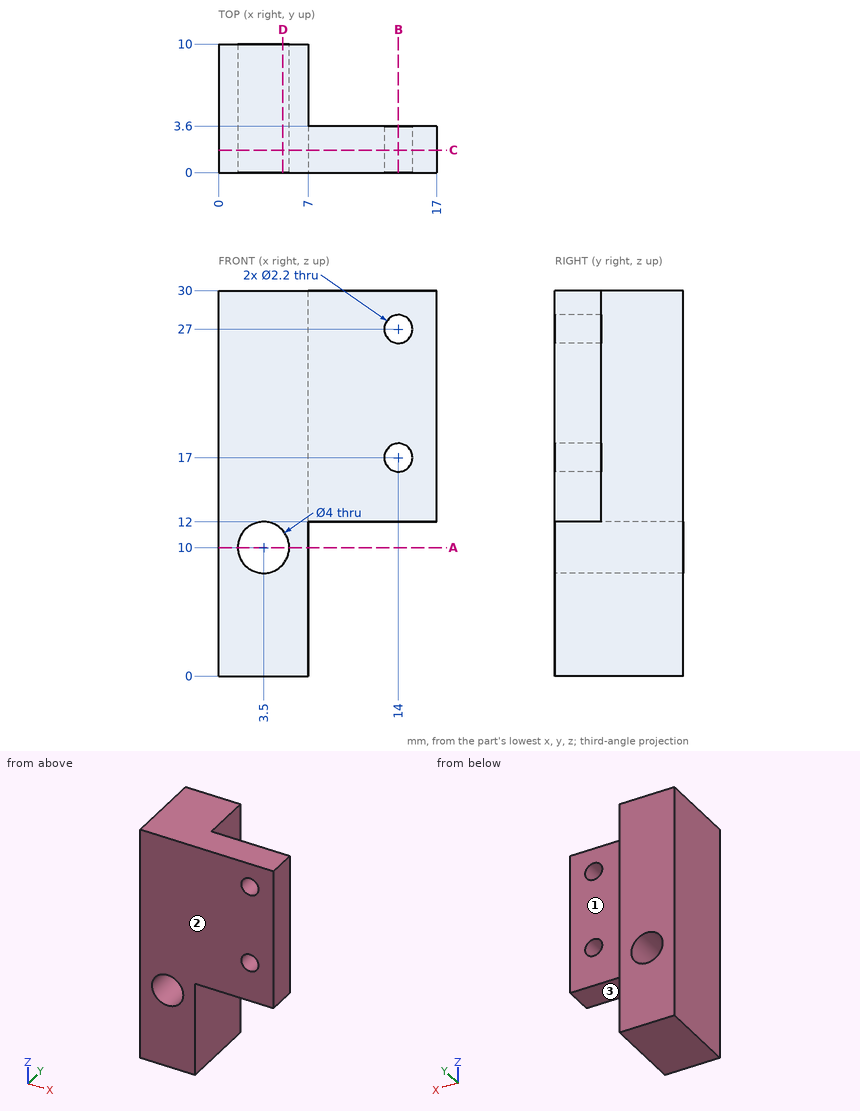
Verification items for this drawing (mm, ordinates from the low corner). A direction names the side the tool comes from. Coordinates: 2 decimals unless noted, no trailing zeros. Order: outer loops, then holes, each group sorted by start corner. A loop starts at its lowest first (then second) coordinate and runs counter-clockwise, first axis right, second up. Notation, with made-up numbers: (-8.75, -11.75) - (28.25, -11.75) arc R31 cw to (28.25, 23.25) - close; hole circle Ø4 at (23.5, 87.5). An arc over 180 degrees is marked (long way). Answer as a JSON object with one key per item and string values. Group by question number.
Item 1: Sectioned sample at D-D, the plane x = 5. Record the cut outline in (y, z), and give its area (3 significant figures).
Item 2: Scan lines: probe 1 along Z at (x, y) = (14, 2.2); probe 2 along Z at (x, y) = (3.5, 5.5); probe 3 along X at (y, z) = (6, 22.75). Record each from-to range of solid material in increasing order.
Item 3: Sectioned sample at C-C, the plane y = 1.75. Record the cut outline in (x, z), and give its area (3 significant figures).
Item 4: Sectioned sample at B-B, the plane x = 14. Record the cut outline in (y, z).
Item 5: Tool access check on the marked faces 1, 2 and 3. Record the directions out of +Z, -Z, +X, -X, +Y, -Y that give a thin tool (end or side, any length) a straight path to the whole face; none if there is none.
Item 6: Depth check by flat-ended pin: pin 1 Ø3.5 at (x, z) = (3.5, 10) entering from +Y; pin 2 Ø4 at (y, z) = (2, 3.5) entering from +X; pin 3 Ø1.8 at (x, y) = (12.5, 2.5) entering from -Z; pin 4 Ø3.5 at (x, z) = (14, 17) entering from +Y. Enter the tip coordinate at first touch or a pass-through.
Item 7: Sectioned sample at A-A, the plane z = 10. Record the cut outline in (x, y).
Resolved:
{
 "1": {"outline": "(0, 0) - (10, 0) - (10, 8.68) - (0, 8.68) - close; (0, 11.32) - (10, 11.32) - (10, 30) - (0, 30) - close", "area": "274 mm^2"},
 "2": {"probe 1": "12 to 15.9, 18.1 to 25.9, 28.1 to 30", "probe 2": "0 to 8, 12 to 30", "probe 3": "0 to 7"},
 "3": {"outline": "(0, 0) - (7, 0) - (7, 12) - (17, 12) - (17, 30) - (0, 30) - close; hole circle Ø4 at (3.5, 10); hole circle Ø2.2 at (14, 17); hole circle Ø2.2 at (14, 27)", "area": "370 mm^2"},
 "4": {"outline": "(0, 12) - (3.6, 12) - (3.6, 15.9) - (0, 15.9) - close; (0, 18.1) - (3.6, 18.1) - (3.6, 25.9) - (0, 25.9) - close; (0, 28.1) - (3.6, 28.1) - (3.6, 30) - (0, 30) - close"},
 "5": {"face 1": "+Z, -Z, +X, +Y", "face 2": "+Z, -Z, +X, -X, -Y", "face 3": "-Z, +X, +Y, -Y"},
 "6": {"pin 1": "through", "pin 2": "x = 7", "pin 3": "z = 12", "pin 4": "y = 3.6"},
 "7": {"outline": "(0, 0) - (1.5, 0) - (1.5, 10) - (0, 10) - close; (5.5, 0) - (7, 0) - (7, 10) - (5.5, 10) - close"}
}
